Input: part model. Units: mm. Frame: model coordinates. Coordinates: 2 decimals unless noted, no trailing zeros. Write each loop counter-clockwise with the first axis right and the second up, starting at its lowest first coordinate (ties: lowest second). Pieces come first, ordered by that corner, then holes.
1) Pin query (flat end, axial travel): pin 1 Ø1.6 at (x, y) = (0, 80) entering from -Z. Return the tip coordinate at first contact, or that it passes through.
2) Section query C-C (x = 0). Output: boundary loops of the cut face in (y, z).
3) Section query A-A (y = 40). Output: boundary loops of the cut face in (x, z).
4) Section query B-B (z = 0.85). Output: boundary loops of the cut face in (x, y).
5) Line query: L1, parallel to Y at x = 0, z = -0.05; L2, parallel to Y at x = 1.5, z = -0.3; L3, parallel to Y at x = -1.75, z = 1.5. Output: solid intervals per line, ascending.
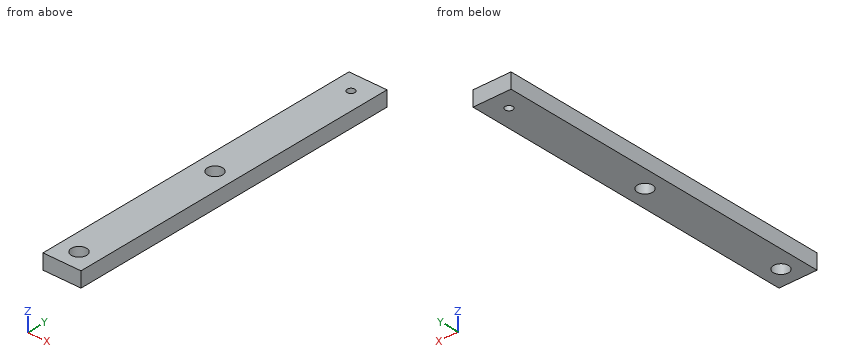
from build123d import *

# Parameters (mm, degrees)
F0_W     = 10
F0_H     = 90
F0_R     = 2
F0_R_2   = 1
F1_DEPTH = 2


with BuildPart() as f1:
    # F0 (on Top) → F1 (new body, symmetric)
    with BuildSketch(Plane.XY):
        with Locations((0, 40)):
            Rectangle(F0_W, F0_H)
        Circle(F0_R, mode=Mode.SUBTRACT)
        with Locations((0, 40)):
            Circle(F0_R, mode=Mode.SUBTRACT)
        with Locations((0, 80)):
            Circle(F0_R_2, mode=Mode.SUBTRACT)
    extrude(amount=F1_DEPTH, both=True)


solid = f1.part
Answer:
1. pin 1: passes through
2. outline: (-5, -2) - (-2, -2) - (-2, 2) - (-5, 2) - close; (2, -2) - (38, -2) - (38, 2) - (2, 2) - close; (42, -2) - (79, -2) - (79, 2) - (42, 2) - close; (81, -2) - (85, -2) - (85, 2) - (81, 2) - close
3. outline: (-5, -2) - (-2, -2) - (-2, 2) - (-5, 2) - close; (2, -2) - (5, -2) - (5, 2) - (2, 2) - close
4. outline: (-5, -5) - (5, -5) - (5, 85) - (-5, 85) - close; hole circle Ø4 at (0, 0); hole circle Ø4 at (0, 40); hole circle Ø2 at (0, 80)
5. L1: y = -5 to -2, 2 to 38, 42 to 79, 81 to 85
5. L2: y = -5 to -1.32, 1.32 to 38.68, 41.32 to 85
5. L3: y = -5 to -0.97, 0.97 to 39.03, 40.97 to 85
